Design review of the part built by this model. Coordinates are the model's own, in mm. A direction names the side the tool comes from. Coordinates: 2 decimals unless noted, no trailing zeros. Write each loop counter-clockwise with the first axis right and the second up, starting at its lowest first coordinate (ties: lowest second). Pieces come first, ordered by that corner, then holes. Notation, with made-up numbers: (89.25, 64) -> (116.25, 64) arc R31 ccw to (116.25, 103) -> close; hole circle Ø7 at (46.25, 73). An arc over 180 degrees is marked (long way). Answer in a Markdown table with one row per item. Add a question column.
Item 1: Take a section at D-D, the plane y = -0.25. Write out the cut boundary in (x, z).
Item 2: Draft analysis for pull direction Z (two halves, no side actions). For faces 1 (the face through (-1.016, -1.887, 0.133)), 2 (the face through (0, -2.8, 0)), state which applies: released by +Z, released by -Z, zero draft, split by the parting line, or undercut.
Item 3: Take a section at C-C, the plane y = -1.55. Write out the cut boundary in (x, z) (3 decimals).
Item 4: Take a section at B-B, the plane z = 0. Write out the cut boundary in (x, y) (3 decimals), and give its area (3 significant figures).
Item 5: Clearance check with a flat-ended pin moving along its axis: P1, Ø1.5, axis at x = 2, z = 0.5, coming from the -Y side. State where the tip first meets the part, or that it passes through.
Item 6: To check wall thickness, follow line 1 (Y direction, x = 2, z = 1); line 2 (X direction, y = -0.35, z = 1.25); line 3 (Z direction, x = -2.25, y = -0.6). State the ranges of each line that lie inside material, in increasing order.
Item 7: For faces 3 (the face through (-1, -1, 1)), 4 (the face through (0, 0, 0)), list the 3-axis set-ups (+Z, -Z, +X, -X, +Y, -Y) from which the entire face can be reached by the end or side of a thin tool; tool diameter is ignored.
Item 8: Take a section at A-A, the plane x = 0. Write out the cut boundary in (y, z) (3 decimals), and give its area (3 significant figures).
from build123d import *


with BuildPart() as part:
    # Эскиз1 → Повернуть1 (revolve)
    with BuildSketch(Plane.XY, mode=Mode.PRIVATE) as revolve_1_sk:
        with BuildLine():
            Line((0, 0), (0, -2.8))
            Line((0, -2.8), (1.025, -2.8))
            Line((1.025, -2.8), (1.025, -1))
            Line((1.025, -1), (2.314086796, -1))
            ThreePointArc((2.314086796, -1), (2.562042805, -0.913875481), (2.703223354, -0.692589088))
            Line((2.703223354, -0.692589088), (2.721726884, -0.614821824))
            ThreePointArc((2.721726884, -0.614821824), (3.004087982, -0.172249038), (3.5, 0))
            Line((3.5, 0), (0, 0))
        make_face()
    revolve(revolve_1_sk.sketch.rotate(Axis((0, 0, 0), (0, 1, 0)), 90), axis=Axis((0, 0, 0), (0, 1, 0)))


solid = part.part
Answers:
| question | item | result |
|---|---|---|
| 1 | outline | circle Ø5.84 at (0, 0) |
| 2 | face 1 | split by the parting line |
| 2 | face 2 | zero draft |
| 3 | outline | circle Ø2.05 at (0, 0) |
| 4 | outline | (-3.5, 0) arc R0.8 cw to (-2.722, -0.615) -> (-2.703, -0.693) arc R0.4 ccw to (-2.314, -1) -> (-1.025, -1) -> (-1.025, -2.8) -> (1.025, -2.8) -> (1.025, -1) -> (2.314, -1) arc R0.4 ccw to (2.703, -0.693) -> (2.722, -0.615) arc R0.8 cw to (3.5, 0) -> close |
| 4 | area | 9.30 mm^2 |
| 5 | P1 | stops at y = -1 |
| 6 | line 1 | y = -1 to 0 |
| 6 | line 2 | x = -2.55 to 2.55 |
| 6 | line 3 | z = -1.54 to 1.54 |
| 7 | face 3 | -Y |
| 7 | face 4 | +Z, -Z, +X, -X, +Y |
| 8 | outline | (-2.8, -1.025) -> (-1, -1.025) -> (-1, -2.314) arc R0.4 ccw to (-0.693, -2.703) -> (-0.615, -2.722) arc R0.8 cw to (0, -3.5) -> (0, 3.5) arc R0.8 cw to (-0.615, 2.722) -> (-0.693, 2.703) arc R0.4 ccw to (-1, 2.314) -> (-1, 1.025) -> (-2.8, 1.025) -> close |
| 8 | area | 9.30 mm^2 |
